Geometry: final body of the model. Coordinates: model frame, mm. A direction names the side the tool comes from. Give positions to 0.01 mm unless a question says otherwise; leave off trailing zeros. Write each loop counter-clockwise with the first axis right and the second up, starting at its lowest first coordinate (ties: lowest second). Pieces come first, ordered by that corner, then holes. Notation, with made-up numbers: (21, 68.5) -> (80, 68.5) arc R36 ccw to (80, 103.5) -> close; hole circle Ø7 at (47, 69.25). An arc over 180 degrees is marked (long way). Use CSV: the item, a comma, the result in double quotes. Start each with the question number.
1) Section C-C (y = -3). Output: boundary loops of the cut face in (x, z), plus the area to 3 significant figures.
2) Material intervals for line 1 (Y direction, x = -1.75, z = -0.15); line 2 (Z direction, x = -1.75, y = -2.25); line 3 (Z direction, x = -9, y = -3), sorted ascending. Write a range as [from, to].
3) Set-up query: faces 1 (the face through (9.65, -0.05, -0.25)), 2 (the face through (1.865, -0.456, -0.746)), 3 (the face through (-9.65, 0.05, -0.25)). Return all of +Z, -Z, +X, -X, +Y, -Y with unobstructed straight access to the full face (end or side cutting, diameter ignored); none if empty.
4) Section A-A (x = 6.25). Output: boundary loops of the cut face in (y, z), plus the area to 4 significant figures.
5) Section B-B (y = 1.5). Output: boundary loops of the cut face in (x, z).
6) Contact query for flat-ended pins moving along their axis: P1, Ø1.5, axis at x = -7.5, z = -1, coming from the -Y side; P2, Ø4, axis at x = 8.5, y = -2, coming from the -Z side. Output: stop coordinate, or through.
7) Draft query along X for faces 4 (the face through (0, 3.85, 1)), 5 (the face through (4.56, 0.03, -0.75)), 6 (the face through (-1.96, -0.29, -0.75)), 7 (the face through (11.15, -0.08, 0.74)). Return one class per face: pulls with the +X half, pulls with the -X half, needs draft (parallel to the pull), parting line crosses it, or undercut.
```python
from build123d import *

# Parameters (mm, degrees)
EXTRUDE_1_DEPTH = 1.5
EXTRUDE_2_DEPTH = 0.5
SKETCH_3_R      = 0.75
EXTRUDE_3_DEPTH = 1
FILLET_2_R      = 0.5


with BuildPart() as part:
    # 草图1 → 凸台-拉伸1 (new body)
    with BuildSketch(Plane.XY):
        with BuildLine():
            Line((7.3, 3.85), (-7.3, 3.85))
            ThreePointArc((-7.3, 3.85), (-11.15, 0), (-7.3, -3.85))
            Line((-7.3, -3.85), (7.3, -3.85))
            ThreePointArc((7.3, -3.85), (11.15, 0), (7.3, 3.85))
        make_face()
    extrude(amount=EXTRUDE_1_DEPTH)

    # 草图2 → 凸台-拉伸2 (add)
    with BuildSketch(Plane(origin=(0, 0, 0), x_dir=(-1, 0, 0), z_dir=(0, 0, -1))):
        with BuildLine():
            Line((-7.35, 2.3), (7.35, 2.3))
            ThreePointArc((7.35, 2.3), (9.65, 0), (7.35, -2.3))
            Line((7.35, -2.3), (-7.35, -2.3))
            ThreePointArc((-7.35, -2.3), (-9.65, 0), (-7.35, 2.3))
        make_face()
    extrude(amount=EXTRUDE_2_DEPTH)

    # 草图3 → 凸台-拉伸3 (add)
    with BuildSketch(Plane(origin=(0, 0, -0.5), x_dir=(-1, 0, 0), z_dir=(0, 0, -1))):
        with Locations((1.27, 0)):
            Circle(SKETCH_3_R)
        with Locations((3.81, 0)):
            Circle(SKETCH_3_R)
        with Locations((-3.81, 0)):
            Circle(SKETCH_3_R)
        with Locations((-1.27, 0)):
            Circle(SKETCH_3_R)
    extrude(amount=EXTRUDE_3_DEPTH)

    # 圆角2
    fillet_2_edges = [part.edges().sort_by_distance(p)[0] for p in [
        (-0.52, 0, -1.5),
        (-3.06, 0, -1.5),
        (4.56, 0, -1.5),
        (2.02, 0, -1.5),
    ]]
    fillet(fillet_2_edges, radius=FILLET_2_R)


solid = part.part
```
Answers follow:
1,outline,"(-9.71, 0) -> (9.71, 0) -> (9.71, 1.5) -> (-9.71, 1.5) -> close"
1,area,"29.1 mm^2"
2,line 1,"y = [-2.3, 2.3]"
2,line 2,"z = [-0.5, 1.5]"
2,line 3,"z = [0, 1.5]"
3,face 1,"-Z, +X"
3,face 2,"-Z"
3,face 3,"-Z, -X"
4,outline,"(-3.85, 0) -> (-2.3, 0) -> (-2.3, -0.5) -> (2.3, -0.5) -> (2.3, 0) -> (3.85, 0) -> (3.85, 1.5) -> (-3.85, 1.5) -> close"
4,area,"13.85 mm^2"
5,outline,"(-10.85, 0) -> (-9.09, 0) -> (-9.09, -0.5) -> (9.09, -0.5) -> (9.09, 0) -> (10.85, 0) -> (10.85, 1.5) -> (-10.85, 1.5) -> close"
6,P1,"stops at y = -2.3"
6,P2,"stops at z = -0.5"
7,face 4,"needs draft"
7,face 5,"undercut"
7,face 6,"undercut"
7,face 7,"pulls with the +X half"
